The model under review builds one solid part; all positions refer to its coordinate system, in mm. Face numbers are marked on the shaded views. A direction names the side the tool comes from. Give positions to 0.01 mm unless a question says otherwise; leave off trailing zeros. Loops run counter-clockwise (first coordinate to the right, second up) from the corner with the lowest first, then second, coordinate; pieces in that order, holes last. Notation, with made-up numbers: (-17.5, 10) - (-0.5, 10) arc R23 cw to (-0.5, 31) - close; hole circle Ø2 at (24.25, 58.5). An arc over 180 degrees is marked (long way). Return JSON: item names as keys, results as strings. Group by question number.
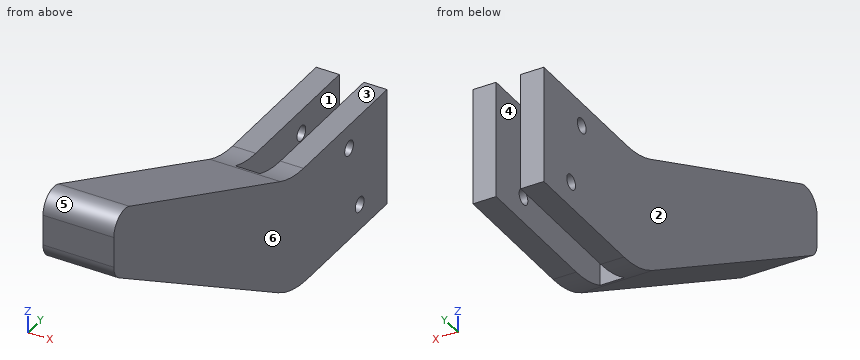
from build123d import *

# Parameters (mm, degrees)
BOSS_EXTRUDE1_DEPTH = 7.5
FILLET1_R           = 20
FILLET2_R           = 4
SKETCH2_W           = 5.2
SKETCH2_H           = 36.194595773
CUT_EXTRUDE1_DEPTH  = 38
CUT_EXTRUDE2_REACH  = 90.345
SKETCH3_R           = 1.6


with BuildPart() as part:
    # Sketch1 → Boss-Extrude1 (new, symmetric)
    with BuildSketch(Plane(origin=(0, 0, 0), x_dir=(0, 0, -1), z_dir=(1, 0, 0))):
        Polygon((-9.803921569, 21.588235294), (15.196078431, 21.588235294), (15.196078431, -13.411764706), (-25.113919349, -78.411764706), (-40.113919349, -78.411764706), (-9.803921569, -13.411764706), align=None)
    extrude(amount=BOSS_EXTRUDE1_DEPTH, both=True)

    # Fillet1
    fillet1_edges = [part.edges().sort_by_distance(p)[0] for p in [
        (0, -13.411764706, -15.196078431),
        (0, -13.411764706, 9.803921569),
    ]]
    fillet(fillet1_edges, radius=FILLET1_R)

    # Fillet2
    fillet2_edges = [part.edges().sort_by_distance(p)[0] for p in [
        (0, -78.411764706, 25.113919349),
        (0, -78.411764706, 40.113919349),
    ]]
    fillet(fillet2_edges, radius=FILLET2_R)

    # Sketch2 → Cut-Extrude1 (cut)
    with BuildSketch(Plane(origin=(0, 21.588235294, 0), x_dir=(1, 0, 0), z_dir=(0, 1, 0))):
        with Locations((0, 1.128729594)):
            Rectangle(SKETCH2_W, SKETCH2_H)
    extrude(amount=-CUT_EXTRUDE1_DEPTH, mode=Mode.SUBTRACT)

    # Cut-Extrude2: up to this face of the body (flat: up to its plane)
    cut_extrude2_end = Plane(part.part.faces().sort_by_distance((7.5, -23.945149467, 6.872044684))[0])
    # Sketch3 → Cut-Extrude2 (cut, up to the picked face)
    with BuildSketch(Plane.ZY.offset(7.5), mode=Mode.PRIVATE) as cut_extrude2_sk1:
        with Locations((-9.696078431, 11.588235294)):
            Circle(SKETCH3_R)
    cut_extrude2_tool1 = split(extrude(cut_extrude2_sk1.sketch, amount=-CUT_EXTRUDE2_REACH, mode=Mode.PRIVATE), bisect_by=cut_extrude2_end, keep=Keep.BOTH, mode=Mode.PRIVATE)
    # Sketch3 → Cut-Extrude2 (cut, up to the picked face)
    with BuildSketch(Plane.ZY.offset(7.5), mode=Mode.PRIVATE) as cut_extrude2_sk2:
        with Locations((4.803921569, 7.702972004)):
            Circle(SKETCH3_R)
    cut_extrude2_tool2 = split(extrude(cut_extrude2_sk2.sketch, amount=-CUT_EXTRUDE2_REACH, mode=Mode.PRIVATE), bisect_by=cut_extrude2_end, keep=Keep.BOTH, mode=Mode.PRIVATE)
    add(cut_extrude2_tool1.solids().sort_by(Axis((-7.5, 11.588235, -9.696078), (1, 0, 0)))[0], mode=Mode.SUBTRACT)
    add(cut_extrude2_tool2.solids().sort_by(Axis((-7.5, 7.702972, 4.803922), (1, 0, 0)))[0], mode=Mode.SUBTRACT)


solid = part.part
Item 1: Mouldability with a two-part tool opening along X and no side actions: class the marked faces 4, 5 and 6 as +X half, -X half, draft (parallel to the pull), parting line (faces both ways), or undercut.
Item 2: Take a section at B-B (z = -3). State the section outline as (x, y) points, then the cut area to 3 significant figures.
Item 3: For L1, parallel to X at y = 17, z = 9.5; L2, parallel to Z at x = 4.5, y = 3; L3, parallel to Y at x = 6.5, z = -8.5, list the stretches that pass through material, from the lowest coordinate up. Write a range as from..to.
Item 4: Take a section at A-A (y = 1). State the section outline as (x, z) points.
Item 5: Tool access review of the marked faces 1, 2 and 3: name each direction out of +Z, -Z, +X, -X, +Y, -Y from which nothing blocks a thin tool from reaching the whole face with its end or side.
Item 6: Take a section at D-D (x = -6.25). State the section outline as (y, z) points.
Item 7: For P1, Ø2.5, axis at x = 5.5, y = 4.5, coming from the +Z side; P2, Ø3, axis at x = 0.5, y = -20.5, coming from the -Z side; P3, Ø6, axis at x = 2, y = -13, coming from the +Z side, all flat-tipped, find the tip position at first contact; note any pin that passes through.
Item 8: Take a section at C-C (x = -1.25). State the section outline as (y, z) points.
Check sheet entries:
{
 "1": {"face 4": "undercut", "face 5": "draft", "face 6": "+X half"},
 "2": {"outline": "(-7.5, -33.08) - (7.5, -33.08) - (7.5, 21.59) - (2.6, 21.59) - (2.6, -16.41) - (-2.6, -16.41) - (-2.6, 21.59) - (-7.5, 21.59) - close", "area": "622 mm^2"},
 "3": {"L1": "x = -7.5..-2.6, 2.6..7.5", "L2": "z = -15.2..9.8", "L3": "y = -24.21..10.53, 12.65..21.59"},
 "4": {"outline": "(-7.5, -15.2) - (-2.6, -15.2) - (-2.6, 9.8) - (-7.5, 9.8) - close; (2.6, -15.2) - (7.5, -15.2) - (7.5, 9.8) - (2.6, 9.8) - close"},
 "5": {"face 1": "+Z, -Z, +Y", "face 2": "+Z, -Z, -X, +Y, -Y", "face 3": "+Z, +X, -X, +Y"},
 "6": {"outline": "(-78.41, 27.34) arc R4 ccw to (-76.52, 23.94) - (-18.25, -12.19) arc R20 ccw to (-7.71, -15.2) - (21.59, -15.2) - (21.59, 9.8) - (-8.98, 9.8) arc R20 cw to (-17.43, 11.68) - (-72.72, 37.46) arc R4 ccw to (-78.41, 33.84) - close; hole circle Ø3.2 at (7.7, 4.8); hole circle Ø3.2 at (11.59, -9.7)"},
 "7": {"P1": "stops at z = 9.8", "P2": "stops at z = -11.73", "P3": "stops at z = 11.05"},
 "8": {"outline": "(-78.41, 27.34) arc R4 ccw to (-76.52, 23.94) - (-18.25, -12.19) arc R20 ccw to (-16.41, -13.21) - (-16.41, 11.24) arc R20 cw to (-17.43, 11.68) - (-72.72, 37.46) arc R4 ccw to (-78.41, 33.84) - close"}
}
